The listing builds one solid part. Answer for the finished solid, in the listing's coordinates (mm). A direction names the side the tool comes from. Round coordinates to 2 decimals unless told otherwise and drop trailing zeros. Write each loop counter-clockwise with the first axis right and the second up, starting at its lowest first coordinate (ties: lowest second). Pieces come first, ordered by that corner, then holes.
(1) For faces 1 (the face through (-79, -58, 2)), 2 (the face through (-1, 1, 7)), 3 (the face through (-79, 58, 2)), determine the directions among +Z, -Z, +X, -X, +Y, -Y from which every point of the face is accessible in a straight line to the end or side of a thin tool.
(2) A cutting plane is placed at A-A, the plane z = 4.25. Give the vertices of the cut face in (x, y), and give its area (3 significant figures).
(3) Find the intervals of material crossed by probe 1 along Y at (x, z) = (29, 2.25), in increasing order.
(4) Each of these flat-tipped pins is pushed along its axis until it touches: pin 1 Ø6.5 at (x, y) = (-79, -58.5) entering from +Z; pin 2 Ø2 at (x, z) = (13, 3.5) entering from +Y; pin 3 Ø2 at (x, z) = (-36.5, 2.5) entering from -Y. Where does it stop, or does it pass through?
(5) A cutting plane is placed at B-B, the plane x = 45.5. Give the vertices of the cut face in (y, z), and give its area (3 significant figures).
from build123d import *

# Parameters (mm, degrees)
F1_DEPTH = 2
F3_DEPTH = 5


with BuildPart() as f1:
    # F0 (on Top) → F1 (new body)
    with BuildSketch(Plane.XY):
        Polygon((82.5, 53.5), (82.5, 62.5), (74.5, 62.5), (74.5, 53.5), (-74.5, 53.5), (-74.5, 62.5), (-82.5, 62.5), (-82.5, 53.5), (-82.5, -53.5), (-82.5, -62.5), (-74.5, -62.5), (-74.5, -53.5), (74.5, -53.5), (74.5, -62.5), (82.5, -62.5), (82.5, -53.5), align=None)
    extrude(amount=F1_DEPTH)

    # F2 (on face) → F3 (join)
    with BuildSketch(Plane.XY.offset(2)):
        Polygon((82.5, -53.5), (82.5, 53.5), (74.5, 53.5), (-74.5, 53.5), (-82.5, 53.5), (-82.5, -53.5), (-74.5, -53.5), (74.5, -53.5), align=None)
    extrude(amount=F3_DEPTH)


solid = f1.part
Solutions:
1. face 1: +Z, +X, -X, -Y
1. face 2: +Z, +X, -X, +Y, -Y
1. face 3: +Z, +X, -X, +Y
2. outline: (-82.5, -53.5) - (82.5, -53.5) - (82.5, 53.5) - (-82.5, 53.5) - close
2. area: 17,700 mm2
3. probe 1: y = -53.5 to 53.5
4. pin 1: stops at z = 2
4. pin 2: stops at y = 53.5
4. pin 3: stops at y = -53.5
5. outline: (-53.5, 0) - (53.5, 0) - (53.5, 7) - (-53.5, 7) - close
5. area: 749 mm2
